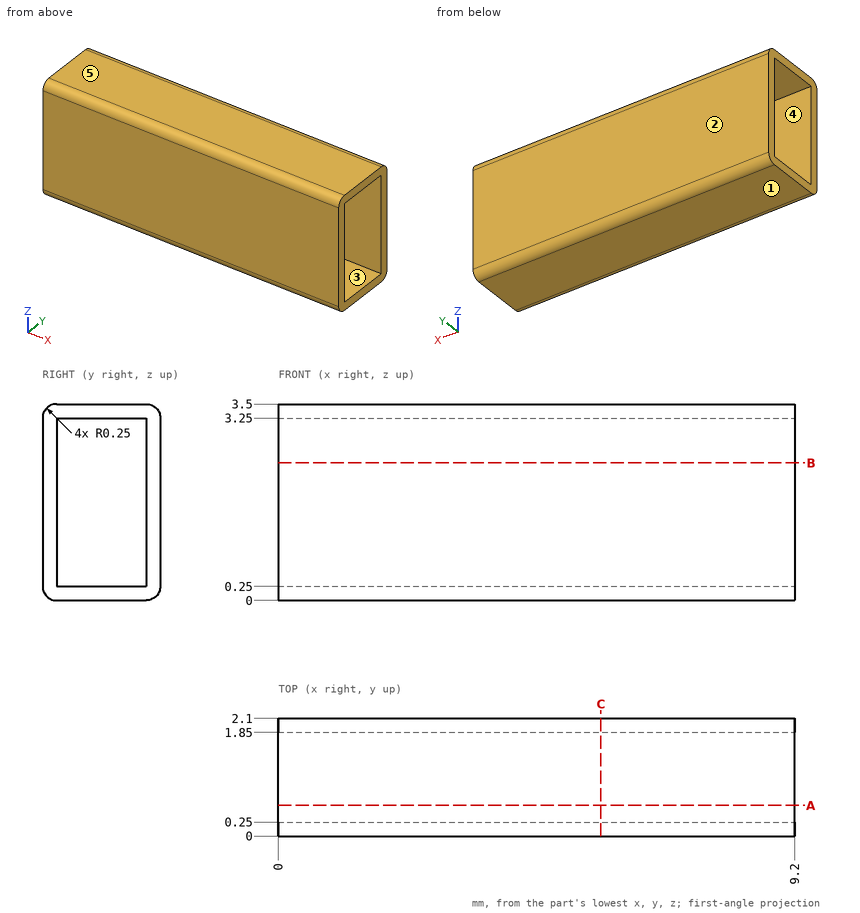
Here's the drawing with two shaded views (mm, measured from the low corner). I have some questions. A direction names the side the tool comes from. Round coordinates to 2 decimals unless told otherwise and drop trailing zeros. Loops run counter-clockwise (first coordinate to the right, second up) from the corner with the lowest first, then second, coordinate; pieces in that order, holes last. Notation, with made-up numbers: (27, -10.75) - (72, -10.75) arc R26 ccw to (72, 7.25) - close; hole circle Ø7 at (47, -20). An arc over 180 degrees is marked (long way). Write item = value, one per line.
1) Imagine slicing it at A-A (y = 0.55). Please give me the cut outline in (x, z), and give its area (3 significant figures).
Computed:
outline = (0, 0) - (9.2, 0) - (9.2, 0.25) - (0, 0.25) - close; (0, 3.25) - (9.2, 3.25) - (9.2, 3.5) - (0, 3.5) - close
area = 4.60 mm2
2) Imagine slicing it at C-C (x = 5.75). Please give me the cut outline in (y, z), and give its area (3 significant figures).
Computed:
outline = (0, 0.25) arc R0.25 ccw to (0.25, 0) - (1.85, 0) arc R0.25 ccw to (2.1, 0.25) - (2.1, 3.25) arc R0.25 ccw to (1.85, 3.5) - (0.25, 3.5) arc R0.25 ccw to (0, 3.25) - close; hole (0.25, 0.25) - (1.85, 0.25) - (1.85, 3.25) - (0.25, 3.25) - close
area = 2.50 mm2
3) If we mould it in two halves opening along Y, with no side actions, what happens to the marked faces 1, 2 and 3? For each: pulls with the +Y half, pulls with the -Y half, needs draft (parallel to the pull), parting line crosses it, or undercut.
Computed:
face_1 = needs draft
face_2 = pulls with the +Y half
face_3 = undercut
4) On a 3-axis mill with a long thin cutter (end or side, diameter ignored), from which of +Z, -Z, +X, -X, +Y, -Y can I reach the whole of each face in a straight line? I mean the marked faces 4 and 5. Say none if no direction works.
Computed:
face_4 = +X, -X
face_5 = +Z, +X, -X, +Y, -Y
5) I need wall thicknesses on line 1 along Y through (x, z) = (6, 2.9); line 2 along Z through (x, y) = (1.25, 0.7); line 3 along Z through (x, y) = (3.25, 0.2). Which ranges of each line are inside material? Lowest first, please. Write a range as from..to.
Computed:
line_1 = 0..0.25, 1.85..2.1
line_2 = 0..0.25, 3.25..3.5
line_3 = 0.01..3.49
6) Imagine slicing it at B-B (z = 2.45). Please give me the cut outline in (x, y).
Computed:
outline = (0, 0) - (9.2, 0) - (9.2, 0.25) - (0, 0.25) - close; (0, 1.85) - (9.2, 1.85) - (9.2, 2.1) - (0, 2.1) - close
